Solid Edge part; units mm, degrees
sketch "Sketch1" plane through (0, 0, 0) normal (0, 0, 1) x (1, 0, 0)
  circle A0 centre (0, 0) radius 7.5
extrude "ExtrudedProtrusion_1" add sketch "Sketch1" along normal blind 250 and the other way blind 85
sketch "Sketch2" plane through (0, 0, 0) normal (0, 0, 1) x (1, 0, 0)
  line L0 (-1.5, 6.5) -> (1.5, 6.5)
  line L1 (1.5, 6.5) -> (1.5, 8.5)
  line L2 (1.5, 8.5) -> (-1.5, 8.5)
  line L3 (-1.5, 8.5) -> (-1.5, 6.5)
  dimension "D1" = 1.5
extrude "ExtrudedProtrusion_2" add sketch "Sketch2" along normal blind 30
sketch "Sketch3" plane through (0, 0, 250) normal (0, 0, 1) x (0, 1, 0)
  line L0 (1.5023, 6.5) -> (-1.5023, 6.5)
  line L1 (-1.5023, 6.5) -> (-1.5023, 8.5)
  line L2 (-1.5023, 8.5) -> (1.5023, 8.5)
  line L3 (1.5023, 8.5) -> (1.5023, 6.5)
  dimension "D1" = 1.5023
  dimension "D2" = 1.5023
extrude "ExtrudedProtrusion_3" add sketch "Sketch3" against normal blind 30
properties material "Aluminum, 1060"
Build history of the part. All positions in model axes, mm. Give positions to 0.01 mm unless a question says otherwise; leave off trailing zeros. Loops run counter-clockwise (first coordinate to the right, second up) from the corner with the lowest first, then second, coordinate; pieces in that order, holes last. Notation, with made-up numbers: (8.5, 55) - (55.5, 55) arc R11 cw to (55.5, 62) - close; hole circle Ø11 at (-19.5, 23.25). An arc over 180 degrees is marked (long way). Write item = value, one per line. Start each with the question number.
1) Band-saw the part on A-A on x = -4.5. Give the cut face in (y, z), plus the area to 3 significant figures.
2) Probe probe 1 along X at (y, z) = (0.5, 2.5); probe 2 along Y at (x, z) = (-0.75, -49); probe 3 along Y at (x, z) = (-1, 43.5). List the from-to ranges inside material, lowest first. Write a range as from..to.
3) Band-saw the part on C-C on z = 123.5. Give the cut face in (x, y), plus the area to 3 significant figures.
4) Drop flat-ended pins along their axis: pin 1 Ø0.9 at (x, z) = (-8, 237.5) entering from -Y; pin 2 Ø1.5 at (y, z) = (-5.5, 15.5) entering from +X; pin 3 Ø2 at (y, z) = (1.5, 145) entering from -X. Give the stop position or say it passes through.
5) Band-saw the part on B-B on z = 6. Give the cut face in (x, y), plus the area to 3 significant figures.
Final values:
q1.outline = (-6, -85) - (6, -85) - (6, 250) - (-6, 250) - close
q1.area = 4,020 mm²
q2.probe_1 = -7.48..7.48
q2.probe_2 = -7.46..7.46
q2.probe_3 = -7.43..7.43
q3.outline = circle Ø15 at (0, 0)
q3.area = 177 mm²
q4.pin_1 = -1.5
q4.pin_2 = 5.8
q4.pin_3 = -7.48
q5.outline = (-1.5, 7.35) arc R7.5 ccw (long way) to (1.5, 7.35) - (1.5, 8.5) - (-1.5, 8.5) - close
q5.area = 180 mm²
